```python
from build123d import *

# Parameters (mm, degrees)
F0_W     = 69.75
F0_H     = 14.75
F1_DEPTH = 40
F2_R     = 2
F4_DEPTH = 14.751
F7_R     = 2


with BuildPart() as f1:
    # F0 (on Top) → F1 (new body)
    with BuildSketch(Plane.XY):
        with Locations((34.875, 0)):
            Rectangle(F0_W, F0_H)
    extrude(amount=F1_DEPTH)

    # F2
    f2_edges = [f1.edges().sort_by_distance(p)[0] for p in [
        (34.875, -7.375, 40),
        (34.875, 7.375, 40),
        (69.75, 0, 40),
        (0, 0, 40),
        (69.75, -7.375, 20),
        (69.75, 7.375, 20),
        (0, -7.375, 20),
        (0, 7.375, 20),
    ]]
    fillet(f2_edges, radius=F2_R)

    # F3 (on face) → F4 (cut, through all)
    with BuildSketch(Plane.XZ.offset(7.375)):
        with BuildLine():
            Line((59.75, 35), (10, 35))
            ThreePointArc((10, 35), (6.464466, 33.535534), (5, 30))
            Line((5, 30), (5, 15))
            ThreePointArc((5, 15), (6.464466, 11.464466), (10, 10))
            Line((10, 10), (59.75, 10))
            ThreePointArc((59.75, 10), (63.285534, 11.464466), (64.75, 15))
            Line((64.75, 15), (64.75, 30))
            ThreePointArc((64.75, 30), (63.285534, 33.535534), (59.75, 35))
        make_face()
    extrude(amount=-F4_DEPTH, mode=Mode.SUBTRACT)

    # F7
    f7_edges = [f1.edges().sort_by_distance(p)[0] for p in [
        (34.875, -7.375, 10),
        (34.875, 7.375, 10),
    ]]
    fillet(f7_edges, radius=F7_R)


solid = f1.part
```
Model file for the job. Use its own axes, mm. A direction names the side the tool comes from. Round coordinates to 2 decimals unless told otherwise and drop trailing zeros. Write each loop counter-clockwise with the first axis right and the second up, starting at its lowest first coordinate (ties: lowest second). Pieces come first, ordered by that corner, then holes. Notation, with made-up numbers: (42, -28.5) -> (94, -28.5) arc R13 ccw to (94, -20.5) -> close; hole circle Ø8 at (43, 47). An arc over 180 degrees is marked (long way). Answer as CSV lines item,"result".
1. Slice it at B-B, the plane x = 39. List the corners of the cut face in (y, z) (3 decimals).
Resolved:
outline,"(-7.375, 0) -> (7.375, 0) -> (7.375, 8) arc R2 ccw to (5.375, 10) -> (-5.375, 10) arc R2 ccw to (-7.375, 8) -> close; (-7.375, 37) arc R2 ccw to (-5.375, 35) -> (5.375, 35) arc R2 ccw to (7.375, 37) -> (7.375, 38) arc R2 ccw to (5.375, 40) -> (-5.375, 40) arc R2 ccw to (-7.375, 38) -> close"
2. Mould opens along X. For faces 6 (the face through (5, 0, 23)), 7 (the face through (0.57, 6.774, 19.266)), 8 (the face through (34, 0, 0)) say: +X half, -X half, draft (parallel to the pull), parting line (faces both ways), or undercut.
Resolved:
face 6,"undercut"
face 7,"-X half"
face 8,"draft"
3. Slice it at C-C, the plane y = 0.25. List the corners of the cut face in (x, z), plus the area to 3 significant figures.
Resolved:
outline,"(0, 0) -> (69.75, 0) -> (69.75, 38) arc R2 ccw to (67.75, 40) -> (2, 40) arc R2 ccw to (0, 38) -> close; hole (5, 15) arc R5 ccw to (10, 10) -> (59.75, 10) arc R5 ccw to (64.75, 15) -> (64.75, 30) arc R5 ccw to (59.75, 35) -> (10, 35) arc R5 ccw to (5, 30) -> close"
area,"1,320 mm²"
4. Tool access for faces 1 (the face through (69.18, 6.774, 19.266)), 2 (the face through (34.527, -6.805, 35.601)), 3 (the face through (6, 0, 12)), 4 (the face through (65.351, 6.805, 22.395)), 5 (the face through (35, -7.375, 5)): list every direction of +Z, -Z, +X, -X, +Y, -Y with a clear straight run to the whole face (end or side of a thin tool).
Resolved:
face 1,"+Z, -Z, +X, +Y"
face 2,"-Y"
face 3,"+Y, -Y"
face 4,"+Y"
face 5,"+Z, -Z, +X, -X, -Y"
5. Slice it at A-A, the plane z = 20. List the corners of the cut face in (x, y) (3 decimals).
Resolved:
outline,"(0, -5.375) arc R2 ccw to (2, -7.375) -> (3, -7.375) arc R2 ccw to (5, -5.375) -> (5, 5.375) arc R2 ccw to (3, 7.375) -> (2, 7.375) arc R2 ccw to (0, 5.375) -> close; (64.75, -5.375) arc R2 ccw to (66.75, -7.375) -> (67.75, -7.375) arc R2 ccw to (69.75, -5.375) -> (69.75, 5.375) arc R2 ccw to (67.75, 7.375) -> (66.75, 7.375) arc R2 ccw to (64.75, 5.375) -> close"
6. Drill centre lines: line 1 (X direction, y = -5, z = 25.5); line 2 (Z direction, x = 22.5, y = -3); line 3 (X direction, y = 5.5, z = 6). Where is each one in solid material? Low to high.
Resolved:
line 1,"0 to 5, 64.75 to 69.75"
line 2,"0 to 10, 35 to 40"
line 3,"0 to 69.75"
